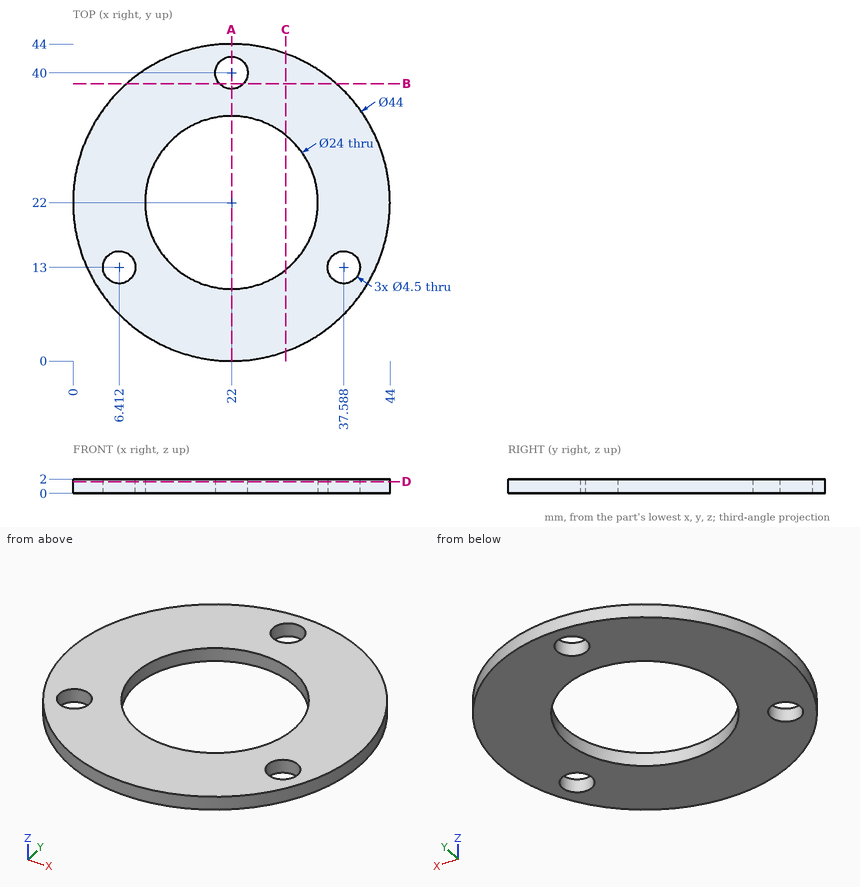
Could you check a few things on this drawing? It's one solid part, dimensions in mm from its lowest x, y, z. Round coordinates to 2 decimals unless told otherwise and drop trailing zeros. Loops run counter-clockwise (first coordinate to the right, second up) from the corner with the lowest first, then second, coordinate; pieces in that order, holes last.
Q1. For P1, Ø3.5, axis at x = 37.59, y = 13, coming from the +Z side, with a flat end and sliding along its axis, tell me the tip position at first contact or that it passes through.
Q2. I want a section at C-C (x = 29.5). Write out the boundary of the cut face in (y, z).
Q3. I want a section at A-A (x = 22). Write out the boundary of the cut face in (y, z).
Q4. I want a section at B-B (y = 38.5). Write out the boundary of the cut face in (x, z).
Q5. I want a section at D-D (z = 1.65). Write out the boundary of the cut face in (x, y), and give its area (3 significant figures).
Q6. Please list where these lines run through material, in increasing order: L1, parallel to Y at x = 22, z = 1.2; L2, parallel to X at y = 13, z = 0.65 (1 decimal); L3, parallel to X at y = 42, z = 1.3 (1 decimal).
Answer below:
1. P1: passes through
2. outline: (1.32, 0) - (12.63, 0) - (12.63, 2) - (1.32, 2) - close; (31.37, 0) - (42.68, 0) - (42.68, 2) - (31.37, 2) - close
3. outline: (0, 0) - (10, 0) - (10, 2) - (0, 2) - close; (34, 0) - (37.75, 0) - (37.75, 2) - (34, 2) - close; (42.25, 0) - (44, 0) - (44, 2) - (42.25, 2) - close
4. outline: (7.45, 0) - (20.32, 0) - (20.32, 2) - (7.45, 2) - close; (23.68, 0) - (36.55, 0) - (36.55, 2) - (23.68, 2) - close
5. outline: circle Ø44 at (22, 22); hole circle Ø4.5 at (6.41, 13); hole circle Ø24 at (22, 22); hole circle Ø4.5 at (22, 40); hole circle Ø4.5 at (37.59, 13)
5. area: 1,020 mm2
6. L1: y = 0 to 10, 34 to 37.75, 42.25 to 44
6. L2: x = 1.9 to 4.2, 8.7 to 14.1, 29.9 to 35.3, 39.8 to 42.1
6. L3: x = 12.8 to 21, 23 to 31.2
